Input: dimensioned drawing with shaded views. Units: mm. Origin: part minimum x, y, z. Round coordinates to 2 decimals unless told otherwise and drop trailing zeros. Order: outer loops, then holes, each group sorted by start corner. A loop starts at its lowest first (then second) coordinate and runs counter-clockwise, first axis right, second up. Notation, with made-up numbers: M 67,89 L 125,89 A7 ccw 125,101 Z; hole C 12.5,81 d5. An arc over 180 degrees is marked long. One line per question, with ' | ' between items.
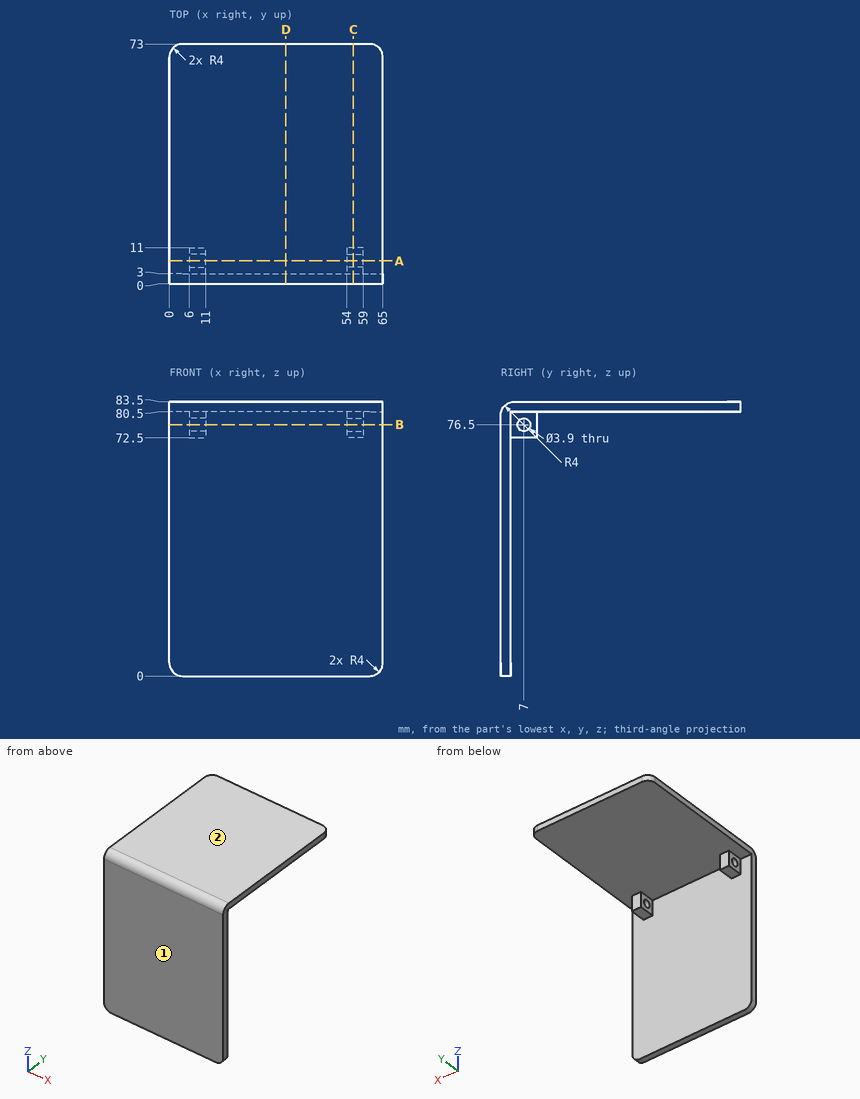
Item 1: First-contact query: pin 1 (2.5 mm diameter, centred on y = 7, z = 76.5, fed in from -X); pin 2 (1.5 mm diameter, centred on x = 7.5, y = 6.5, fed in from -Z); pin 3 (19.5 mm diameter, centred on x = 27.5, z = 43.5, fed in from +Y); pin 4 (10 mm diameter, centred on x = 44.5, y = 41.5, fed in from -Z). Flat tips, straight axial feed; report the tip coordinate or a pass-through.
Report:
pin 1: through | pin 2: z = 72.5 | pin 3: y = 3 | pin 4: z = 80.5
Item 2: Section query B-B, the plane z = 76.5. Return loops of the section in (x, y), plus the area to 3 significant figures.
Report:
outline: M 0,0 L 65,0 L 65,3 L 59,3 L 59,5.05 L 54,5.05 L 54,3 L 11,3 L 11,5.05 L 6,5.05 L 6,3 L 0,3 Z; M 6,8.95 L 11,8.95 L 11,11 L 6,11 Z; M 54,8.95 L 59,8.95 L 59,11 L 54,11 Z | area: 236 mm²
Item 3: Line query: line 1 along Z through (x, y) = (57, 7); line 2 along Y through (x, z) = (22, 67.5); line 3 along Z through (x, y) = (44, 5). Output: solid intervals per line, ascending. Write a range as from..to.
Report:
line 1: 72.5..74.55, 78.45..83.5 | line 2: 0..3 | line 3: 80.5..83.5
Item 4: Section query A-A, the plane y = 7. Return loops of the section in (x, z), plus the area to 3 significant figures.
Report:
outline: M 0,80.5 L 6,80.5 L 6,78.45 L 11,78.45 L 11,80.5 L 54,80.5 L 54,78.45 L 59,78.45 L 59,80.5 L 65,80.5 L 65,83.5 L 0,83.5 Z; M 6,72.5 L 11,72.5 L 11,74.55 L 6,74.55 Z; M 54,72.5 L 59,72.5 L 59,74.55 L 54,74.55 Z | area: 236 mm²
Item 5: Section query C-C, the plane x = 56. Return loops of the section in (y, z).
Report:
outline: M 0,0 L 3,0 L 3,72.5 L 11,72.5 L 11,80.5 L 73,80.5 L 73,83.5 L 4,83.5 A4 ccw 0,79.5 Z; hole C 7,76.5 d3.9
Item 6: Section query D-D, the plane x = 35.5. Return loops of the section in (y, z).
Report:
outline: M 0,0 L 3,0 L 3,80.5 L 73,80.5 L 73,83.5 L 4,83.5 A4 ccw 0,79.5 Z
Item 7: Mould query, pull axis Z, two halves, no side actions, for the marked faces 1 and 2. Classes: +Z half, -Z half, draft (parallel to the pull), parting line (faces both ways), or undercut.
Report:
face 1: draft | face 2: +Z half
